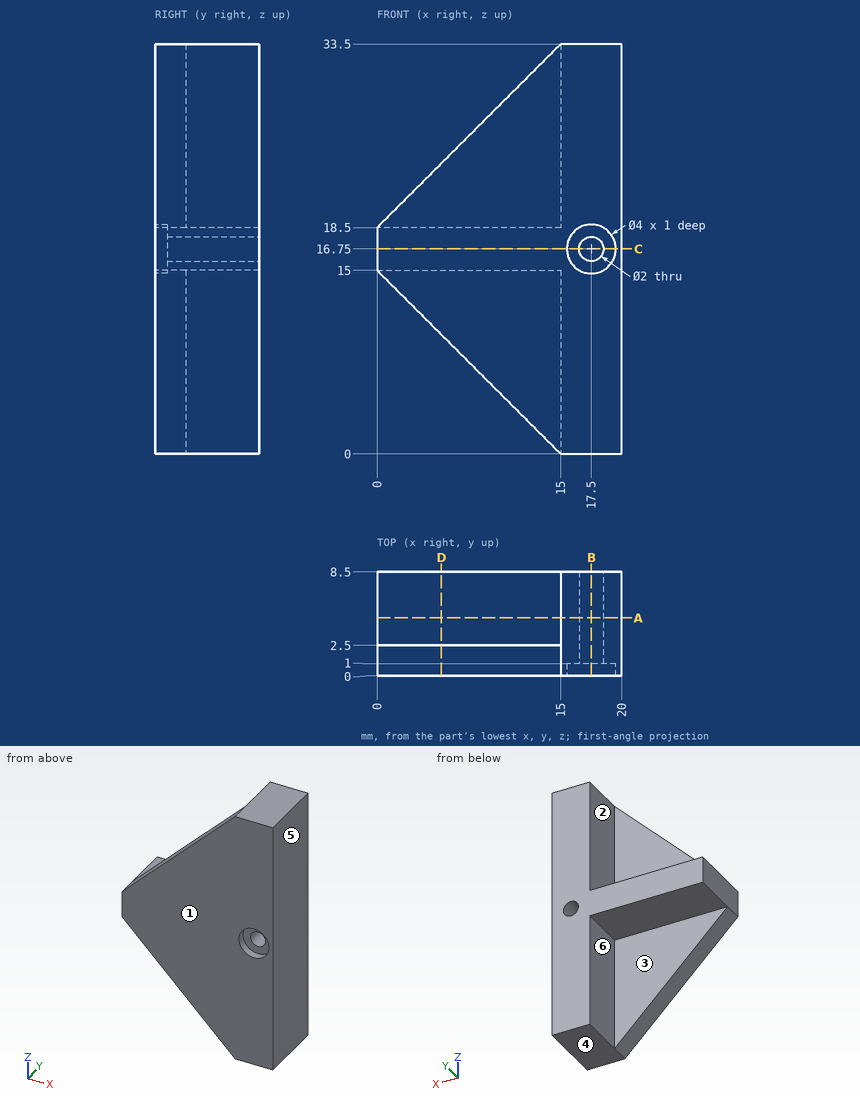
Study the drawing (mm; zero at the part's minimum x, y, z) and answer. A direction names the side the tool comes from. Coordinates: 2 decimals unless noted, no trailing zeros. Loops run counter-clockwise (first coordinate to the right, second up) from the corner with the lowest first, then second, coordinate; pieces in that order, holes last. Notation, with made-up numbers: (-38.75, -40) -> (-25.75, -40) arc R13 cw to (-25.75, -23) -> close; hole circle Ø6 at (19.25, -23.5). An arc over 180 degrees is marked (long way). Write item = value, one per line. Start each with the question number.
1) The part is cut by section B-B, the plane x = 17.5. Determine the outline of the cut face in (y, z).
2) Given P1, Ø3, axis at x = 8, y = 6.5, coming from the +Z side; P2, Ø5, axis at y = 4.5, z = 24, coming from the -X side; P3, Ø3, axis at y = 6, z = 5, coming from the -X side, each flat-ended and moving along its own axis, determine where each tip first touches the part or whether it passes through.
3) The mould has two halves that part along X. Classify the marked faces 4, 5 and 6: pulls with the +X half, pulls with the -X half, needs draft (parallel to the pull), parting line crosses it, or undercut.
4) For the marked faces 1, 2 and 3, determine the directions among +Z, -Z, +X, -X, +Y, -Y from which every point of the face is accessible in a straight line to the end or side of a thin tool.
5) Find the intervals of material crossed by L1, parallel to Z at x = 17.5, y = 3.25; L2, parallel to Z at x = 17.5, y = 0.8; L3, parallel to Y at x = 10.5, z = 8, in increasing order. Write a range as from..to.
6) The part is cut by section C-C, the plane z = 16.75. Determine the outline of the cut face in (x, y).
7) The part is cut by section D-D, the plane x = 5.25. Determine the outline of the cut face in (y, z), plus the area to 3 significant figures.
8) The part is cut by section A-A, the plane y = 4.75. Determine the outline of the cut face in (x, z).
Result:
q1.outline = (0, 0) -> (8.5, 0) -> (8.5, 15.75) -> (1, 15.75) -> (1, 14.75) -> (0, 14.75) -> close; (0, 18.75) -> (1, 18.75) -> (1, 17.75) -> (8.5, 17.75) -> (8.5, 33.5) -> (0, 33.5) -> close
q2.P1 = 18.5
q2.P2 = 4
q2.P3 = 15
q3.face_4 = needs draft
q3.face_5 = pulls with the +X half
q3.face_6 = pulls with the -X half
q4.face_1 = +Z, -Z, +X, -X, -Y
q4.face_2 = +Z, -X, +Y
q4.face_3 = -Z, -X, +Y
q5.L1 = 0..15.75, 17.75..33.5
q5.L2 = 0..14.75, 18.75..33.5
q5.L3 = 0..2.5
q6.outline = (0, 0) -> (15.5, 0) -> (15.5, 1) -> (16.5, 1) -> (16.5, 8.5) -> (0, 8.5) -> close; (18.5, 1) -> (19.5, 1) -> (19.5, 0) -> (20, 0) -> (20, 8.5) -> (18.5, 8.5) -> close
q7.outline = (0, 9.75) -> (2.5, 9.75) -> (2.5, 15) -> (8.5, 15) -> (8.5, 18.5) -> (2.5, 18.5) -> (2.5, 23.75) -> (0, 23.75) -> close
q7.area = 56.0 mm²
q8.outline = (0, 15) -> (15, 15) -> (15, 0) -> (20, 0) -> (20, 33.5) -> (15, 33.5) -> (15, 18.5) -> (0, 18.5) -> close; hole circle Ø2 at (17.5, 16.75)
